```python
from build123d import *

# Parameters (mm, degrees)
SKETCH_1_W           = 20
SKETCH_1_H           = 20
EXTRUDE_1_DEPTH      = 120
SKETCH_2_W           = 10
SKETCH_2_H           = 20
CUT_EXTRUDE_1_DEPTH  = 120
CUT_EXTRUDE_2_DEPTH  = 120
SKETCH_4_R           = 3
CUT_EXTRUDE_3_DEPTH  = 2
SKETCH_6_R           = 1.49
CUT_EXTRUDE_4_DEPTH  = 20
CUT_EXTRUDE_5_DEPTH  = 20
SKETCH_8_W           = 19.6
SKETCH_8_H           = 0.2
SKETCH_8_W_2         = 0.2
SKETCH_8_H_2         = 19.6
CUT_EXTRUDE_6_DEPTH  = 45
EXTRUDE_2_DEPTH      = 24.8
EXTRUDE_START        = 5.2
EXTRUDE_3_DEPTH      = 5.2
SKETCH_12_W          = 20
SKETCH_12_H          = 20
EXTRUDE_4_DEPTH      = 15
CUT_EXTRUDE_7_DEPTH  = 15
SKETCH_14_R          = 2
CUT_EXTRUDE_8_DEPTH  = 70
SKETCH_15_R          = 1.5
CUT_EXTRUDE_9_DEPTH  = 5
SKETCH_16_R          = 3
CUT_EXTRUDE_10_DEPTH = 2
CUT_EXTRUDE_11_DEPTH = 20
SKETCH_18_W          = 0.2
SKETCH_18_H          = 25.5
CUT_EXTRUDE_12_DEPTH = 15


with BuildPart() as part:
    # 草图1 → 凸台-拉伸1 (new body)
    with BuildSketch(Plane.XY):
        with Locations((10, 10)):
            Rectangle(SKETCH_1_W, SKETCH_1_H)
    extrude(amount=EXTRUDE_1_DEPTH)

    # 草图2 → 切除-拉伸1 (cut)
    with BuildSketch(Plane(origin=(0, 20, 0), x_dir=(1, 0, 0), z_dir=(0, 1, 0))):
        with Locations((15, -10)):
            Rectangle(SKETCH_2_W, SKETCH_2_H)
    extrude(amount=-CUT_EXTRUDE_1_DEPTH, mode=Mode.SUBTRACT)

    # 草图3 → 切除-拉伸2 (cut)
    with BuildSketch(Plane(origin=(10, 0, 0), x_dir=(0, 0, -1), z_dir=(1, 0, 0))):
        with BuildLine():
            ThreePointArc((-8.45, 10), (-9.40684068, 11.432013275), (-11.096015511, 11.096015511))
            Line((-11.096015511, 11.096015511), (-8.903984489, 8.903984489))
            ThreePointArc((-8.903984489, 8.903984489), (-8.567986725, 9.40684068), (-8.45, 10))
        make_face()
        with BuildLine():
            Line((-8.903984489, 8.903984489), (-11.096015511, 11.096015511))
            ThreePointArc((-11.096015511, 11.096015511), (-11.096015511, 8.903984489), (-8.903984489, 8.903984489))
        make_face()
    extrude(amount=-CUT_EXTRUDE_2_DEPTH, mode=Mode.SUBTRACT)

    # 草图4 → 切除-拉伸3 (cut)
    with BuildSketch(Plane.ZY):
        with Locations((10, 10)):
            Circle(SKETCH_4_R)
    extrude(amount=-CUT_EXTRUDE_3_DEPTH, mode=Mode.SUBTRACT)

    # 草图6 → 切除-拉伸4 (cut)
    with BuildSketch(Plane.ZY):
        with Locations((92.5, 10)):
            Circle(SKETCH_6_R)
    extrude(amount=-CUT_EXTRUDE_4_DEPTH, mode=Mode.SUBTRACT)

    # 草图7 → 切除-拉伸5 (cut)
    with BuildSketch(Plane.XZ):
        with BuildLine():
            ThreePointArc((11.55, 97.5), (10.844615988, 98.799662969), (9.370485378, 98.9164079))
            Line((9.370485378, 98.9164079), (10.629514622, 96.0835921))
            ThreePointArc((10.629514622, 96.0835921), (11.299662969, 96.655384012), (11.55, 97.5))
        make_face()
        with BuildLine():
            Line((10.629514622, 96.0835921), (9.370485378, 98.9164079))
            ThreePointArc((9.370485378, 98.9164079), (8.5835921, 96.870485378), (10.629514622, 96.0835921))
        make_face()
    extrude(amount=-CUT_EXTRUDE_5_DEPTH, mode=Mode.SUBTRACT)

    # 草图8 → 切除-拉伸6 (cut)
    with BuildSketch(Plane.XY.offset(120)):
        with Locations((10, 19.9)):
            Rectangle(SKETCH_8_W, SKETCH_8_H)
        with Locations((0.1, 19.9)):
            Rectangle(SKETCH_8_W_2, SKETCH_8_H)
        with Locations((0.1, 10)):
            Rectangle(SKETCH_8_W_2, SKETCH_8_H_2)
        with Locations((19.9, 10)):
            Rectangle(SKETCH_8_W_2, SKETCH_8_H_2)
        with Locations((19.9, 0.1)):
            Rectangle(SKETCH_8_W_2, SKETCH_8_H)
        with Locations((10, 0.1)):
            Rectangle(SKETCH_8_W, SKETCH_8_H)
        with Locations((0.1, 0.1)):
            Rectangle(SKETCH_8_W_2, SKETCH_8_H)
        with Locations((19.9, 19.9)):
            Rectangle(SKETCH_8_W_2, SKETCH_8_H)
    extrude(amount=-CUT_EXTRUDE_6_DEPTH, mode=Mode.SUBTRACT)

    # 草图9 → 凸台-拉伸2 (add)
    with BuildSketch(Plane(origin=(0, 19.8, 0), x_dir=(1, 0, 0), z_dir=(0, 1, 0))):
        with BuildLine():
            Line((0, -75), (-10, -75))
            ThreePointArc((-10, -75), (-2.928932188, -77.928932188), (0, -85))
            Line((0, -85), (0.2, -85))
            Line((0.2, -85), (0.2, -75))
            Line((0.2, -75), (0, -75))
        make_face()
    extrude(amount=-EXTRUDE_2_DEPTH)

    # 草图10 → 凸台-拉伸3 (add)
    with BuildSketch(Plane(origin=(0, 19.8, 0), x_dir=(1, 0, 0), z_dir=(0, 1, 0)).offset(EXTRUDE_START)):
        with BuildLine():
            Line((-10, -75), (0, -75))
            Line((0, -75), (0.2, -75))
            Line((0.2, -75), (0.2, -85))
            Line((0.2, -85), (0, -85))
            ThreePointArc((0, -85), (-2.928932188, -77.928932188), (-10, -75))
        make_face()
    extrude(amount=-EXTRUDE_3_DEPTH)

    # 草图12 → 凸台-拉伸4 (add)
    with BuildSketch(Plane(origin=(0, 20, 0), x_dir=(1, 0, 0), z_dir=(0, 1, 0))):
        with Locations((10, -65)):
            Rectangle(SKETCH_12_W, SKETCH_12_H)
    extrude(amount=EXTRUDE_4_DEPTH)

    # 草图13 → 切除-拉伸7 (cut)
    with BuildSketch(Plane.ZY):
        Polygon((65, 20), (60, 20), (60, 4), (70, 4), (70, 20), align=None)
        Polygon((60, 29.5), (60, 20), (65, 20), (65, 25), (65, 29.5), align=None)
        Polygon((65, 25), (65, 20), (70, 20), (70, 29.5), (65, 29.5), align=None)
    extrude(amount=-CUT_EXTRUDE_7_DEPTH, mode=Mode.SUBTRACT)

    # 草图14 → 切除-拉伸8 (cut)
    with BuildSketch(Plane(origin=(0, 0, 0), x_dir=(-1, 0, 0), z_dir=(0, 0, -1))):
        with Locations((-5, 6)):
            Circle(SKETCH_14_R)
    extrude(amount=-CUT_EXTRUDE_8_DEPTH, mode=Mode.SUBTRACT)

    # 草图15 → 切除-拉伸9 (cut)
    with BuildSketch(Plane.ZY.offset(-15)):
        with Locations((65, 14.5)):
            Circle(SKETCH_15_R)
    extrude(amount=-CUT_EXTRUDE_9_DEPTH, mode=Mode.SUBTRACT)

    # 草图16 → 切除-拉伸10 (cut)
    with BuildSketch(Plane(origin=(20, 0, 0), x_dir=(0, 0, -1), z_dir=(1, 0, 0))):
        with Locations((-65, 14.5)):
            Circle(SKETCH_16_R)
    extrude(amount=-CUT_EXTRUDE_10_DEPTH, mode=Mode.SUBTRACT)

    # 草图17 → 切除-拉伸11 (cut)
    with BuildSketch(Plane.ZY):
        with BuildLine():
            Line((60, 35), (55, 35))
            Line((55, 35), (55, 30))
            ThreePointArc((55, 30), (56.464466094, 33.535533906), (60, 35))
        make_face()
        with BuildLine():
            Line((75, 35), (70, 35))
            ThreePointArc((70, 35), (73.535533906, 33.535533906), (75, 30))
            Line((75, 30), (75, 35))
        make_face()
    extrude(amount=-CUT_EXTRUDE_11_DEPTH, mode=Mode.SUBTRACT)

    # 草图18 → 切除-拉伸12 (cut)
    with BuildSketch(Plane.ZY):
        with Locations((59.9, 16.75)):
            Rectangle(SKETCH_18_W, SKETCH_18_H)
        Polygon((70, 29.5), (70.2, 29.5), (70.2, 29.7), (59.8, 29.7), (59.8, 29.5), (60, 29.5), align=None)
        with Locations((70.1, 16.75)):
            Rectangle(SKETCH_18_W, SKETCH_18_H)
    extrude(amount=-CUT_EXTRUDE_12_DEPTH, mode=Mode.SUBTRACT)


solid = part.part
```
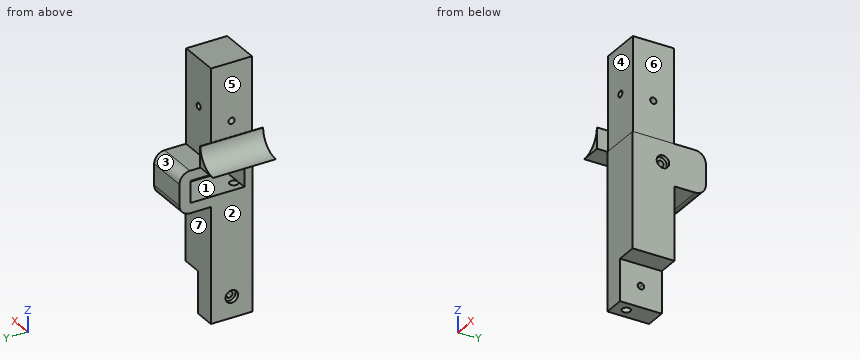
Geometry check sheet. Reference: the model listing, model coordinates, mm. Face numbers are marked on the shaded views. A direction names the side the tool comes from. Coordinates: 2 decimals unless noted, no trailing zeros. Loops run counter-clockwise (first coordinate to the right, second up) from the corner with the lowest first, then second, coordinate; pieces in that order, holes last. Notation, with made-up numbers: (-28.5, 74) - (9.5, 74) arc R10 cw to (9.5, 83) - close; hole circle Ø1 at (-24.5, -28). An arc over 180 degrees is marked (long way). One line per item, written item: value. Start each with the question number.
(1) Cross-section at C-C on y = 23. Enter the section's corners in (x, z), plus the area to 3 significant figures.
(2) Depth check by flat-ended pin: P1, Ø8, axis at x = 6.5, y = 29, coming from the -Z side; P2, Ø10, axis at y = 9.5, z = 101, coming from the -X side; P3, Ø3, axis at y = 22, z = 66, coming from the -X side. Enter the tip coordinate at first touch or a pass-through.
(3) Cross-section at A-A on z = 92.5. Enter the section's corners in (x, y).
(4) Cross-section at B-B on y = 28.5. Enter the section's corners in (x, z), plus the area to 3 significant figures.
(5) Material ranges on line 1 (Y direction, x = 5, z = 92.5); line 2 (X direction, y = 6, z = 25); line 3 (Z direction, x = 2.5, y = 5), recorded low to high. Write a range as [from, to].
(6) Mould release check, pull along Z, two halves, no side actions. Record for the marked faces 1, 2 and 3: released by +Z, released by -Z, zero draft, split by the parting line, or undercut.
(7) Tool access check on the marked faces 4, 5, 6 and 7. Record the directions out of +Z, -Z, +X, -X, +Y, -Y that give a thin tool (end or side, any length) a straight path to the whole face; none if there is none.
(8) Cross-section at D-D on z = 78. Enter the section's corners in (x, y), plus the area to 3 significant figures.
Results below:
1. outline: (-10, 75) - (0, 75) - (0, 70.2) - (15, 70.2) - (15, 59.8) - (0, 59.8) - (0, 55) - (20, 55) - (20, 75) - (0.2, 75) - (0.2, 85) - (0, 85) arc R10 cw to start
1. area: 267 mm2
2. P1: stops at z = 55
2. P2: stops at x = 0.2
2. P3: stops at x = 15
3. outline: (0.2, 0.2) - (19.8, 0.2) - (19.8, 8.51) - (0.2, 8.51) - close; (0.2, 11.49) - (19.8, 11.49) - (19.8, 19.8) - (0.2, 19.8) - close
4. outline: (0, 55) - (20, 55) - (20, 75) - (0, 75) - (0, 70.2) - (15, 70.2) - (15, 59.8) - (0, 59.8) - close
4. area: 244 mm2
5. line 1: y = [0.2, 8.51], [11.49, 19.8]
5. line 2: x = [0, 3], [7, 20]
5. line 3: z = [0, 59.8], [70.2, 120]
6. face 1: undercut
6. face 2: zero draft
6. face 3: released by +Z
7. face 4: +Z, +X, -Y
7. face 5: +Z, -X, +Y, -Y
7. face 6: +Z, +X, +Y, -Y
7. face 7: -Z, +X, -X, +Y
8. outline: (-2.86, -5) - (0.2, -5) - (0.2, 0.2) - (19.8, 0.2) - (19.8, 19.8) - (0.2, 19.8) - (0.2, 25) - (-2.86, 25) - close
8. area: 476 mm2
